Part model, mm, in its own coordinate system. A direction names the side the tool comes from. Coordinates: 2 decimals unless noted, no trailing zeros. Order: outer loops, then holes, each group sorted by start corner. A loop starts at its lowest first (then second) coordinate and runs counter-clockwise, first axis right, second up.
1) Wall check: L1, parallel to Y at x = -76.5, z = -12; L2, parallel to X at y = 8.25, z = -102.5. Give the ranges that are in metal, low to high.
2) Pin check, flat tips, straight feed: pin 1 Ø7.5 at (y, z) = (7.5, 72) entering from +X; pin 2 Ø0.9 at (y, z) = (1.5, 7) entering from -X; pin 3 Ø10 at (x, y) = (135.5, 9) entering from +Z; pin 4 Ø4 at (y, z) = (12.5, 64.5) entering from -X. Stop position of each tip, or through.
3) Mould opens along Y. For faces 4 (the flat face through (3, 10, 2)), 5 (the flat face through (-3, 0, -2)), 6 (the cylindrical face through (0.04, 14.99, -142.15)) say: +Y half, -Y half, draft (parallel to the pull), parting line (faces both ways), or undercut.
4) Cut at B-B (z = 87). List the corners of the cut face in (x, y).
5) Cut at C-C (y = 13). List the corners of the cut face in (x, z).
6) Cut at A-A (x = -130). List the corners of the cut face in (y, z).
7) Tool access for faces 1 (the flat face through (-3, 10, 2)), 2 (the flat face through (124.8, 3, -2)), 3 (the cylindrical face through (0.04, 14.99, 142.15)): list every direction of +Z, -Z, +X, -X, +Y, -Y with a clear straight run to the whole face (end or side of a thin tool).
```python
from build123d import *

# Parameters (mm, degrees)
BOSS_EXTRUDE1_DEPTH = 3
SKETCH2_W           = 10
SKETCH2_H           = 30
CUT_EXTRUDE1_DEPTH  = 3
SKETCH3_W           = 6
SKETCH3_H           = 290
BOSS_EXTRUDE2_DEPTH = 15
FILLET1_R           = 10


with BuildPart() as part:
    # Sketch1 → Boss-Extrude1 (new body)
    with BuildSketch(Plane(origin=(0, 0, 0), x_dir=(1, 0, 0), z_dir=(0, 1, 0))):
        Polygon((-250, -145), (250, -145), (250, 145), (-250, 145), (-250, 70), (-215, 70), (-215, -23), (-250, -23), align=None)
    extrude(amount=BOSS_EXTRUDE1_DEPTH)

    # Sketch2 → Cut-Extrude1 (cut)
    with BuildSketch(Plane(origin=(0, 3, 0), x_dir=(1, 0, 0), z_dir=(0, 1, 0))):
        with Locations((130, 0)):
            Rectangle(SKETCH2_W, SKETCH2_H)
        with Locations((-130, 0)):
            Rectangle(SKETCH2_W, SKETCH2_H)
    extrude(amount=-CUT_EXTRUDE1_DEPTH, mode=Mode.SUBTRACT)

    # Sketch3 → Boss-Extrude2 (add)
    with BuildSketch(Plane(origin=(0, 3, 0), x_dir=(1, 0, 0), z_dir=(0, 1, 0))):
        Rectangle(SKETCH3_W, SKETCH3_H)
    extrude(amount=BOSS_EXTRUDE2_DEPTH)

    # Fillet1
    fillet1_edges = [part.edges().sort_by_distance(p)[0] for p in [
        (0, 18, -145),
        (0, 18, 145),
    ]]
    fillet(fillet1_edges, radius=FILLET1_R)


solid = part.part
```
Geometry check:
1. L1: y = 0 to 3
1. L2: x = -3 to 3
2. pin 1: stops at x = 3
2. pin 2: stops at x = -215
2. pin 3: passes through
2. pin 4: stops at x = -3
3. face 4: draft
3. face 5: -Y half
3. face 6: +Y half
4. outline: (-250, 0) - (250, 0) - (250, 3) - (3, 3) - (3, 18) - (-3, 18) - (-3, 3) - (-250, 3) - close
5. outline: (-3, -143.66) - (3, -143.66) - (3, 143.66) - (-3, 143.66) - close
6. outline: (0, -145) - (3, -145) - (3, -15) - (0, -15) - close; (0, 15) - (3, 15) - (3, 145) - (0, 145) - close
7. face 1: +Z, -Z, -X, +Y
7. face 2: +Z, -Z, +X, +Y
7. face 3: +Z, +X, -X, +Y
